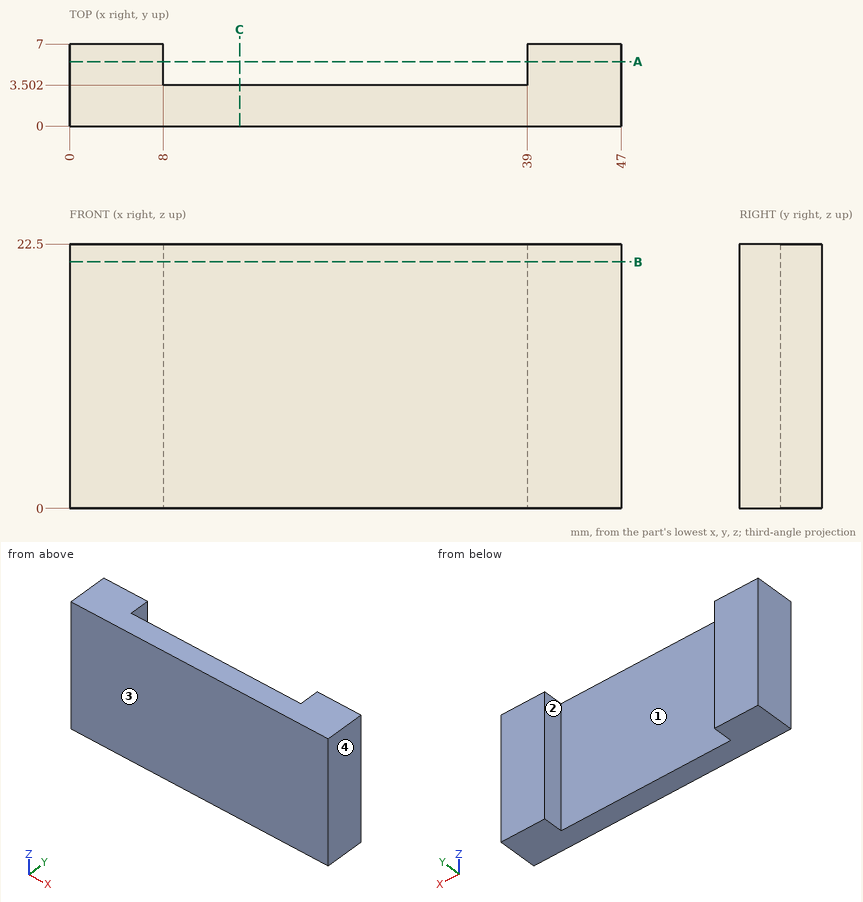
Design review of the part shown in the three views and the two pictorial views. Dimensions are in mm from the part's minimum x, y and z. Give positions to 0.01 mm unless a question says otherwise; leave off trailing zeros. Write each loop counter-clockwise with the first axis right and the second up, starting at its lowest first coordinate (ties: lowest second). Pieces come first, ordered by that corner, then holes.
Item 1: Insertion check: P1, Ø1.5, axis at x = 23.5, z = 20, coming from the +Y side. The pin has a flat end and moves straight along its axis. Give the tip position at first contact, or say it passes through.
Item 2: The part is to be moulded in two halves that separate along X. For the marked faces 1, 2, 3 and 4, say which applies: +X half, -X half, draft (parallel to the pull), parting line (faces both ways), or undercut.
Item 3: Wall thickness on probe 1 along X at (y, z) = (6.25, 19); probe 2 along Y at (x, z) = (37.5, 18): over which ranges is each line inside the solid? List them lowest first.
Item 4: Take a section at A-A (y = 5.5). Give the boundary of the cut face in (x, z).
Item 5: Take a section at B-B (z = 21). Give the boundary of the cut face in (x, y).
Item 6: Take a section at C-C (x = 14.5). Give the boundary of the cut face in (y, z), and give its area (3 significant figures).
Established:
1. P1: stops at y = 3.5
2. face 1: undercut
2. face 2: undercut
2. face 3: draft
2. face 4: +X half
3. probe 1: x = 0 to 8, 39 to 47
3. probe 2: y = 0 to 3.5
4. outline: (0, 0) - (8, 0) - (8, 22.5) - (0, 22.5) - close; (39, 0) - (47, 0) - (47, 22.5) - (39, 22.5) - close
5. outline: (0, 0) - (47, 0) - (47, 7) - (39, 7) - (39, 3.5) - (8, 3.5) - (8, 7) - (0, 7) - close
6. outline: (0, 0) - (3.5, 0) - (3.5, 22.5) - (0, 22.5) - close
6. area: 78.8 mm2
